Here's how the part is built. I have some questions about the finished solid (model axes, mm). A direction names the side the tool comes from. Give positions to 0.01 mm unless a question says otherwise; leave off trailing zeros. Loops run counter-clockwise (first coordinate to the right, second up) from the corner with the lowest first, then second, coordinate; pieces in that order, holes last.
Q1. Thinking about a two-plate mould opening in X: for faces 6 (the face through (-114, 50, -1)), 7 (the face through (111.01, 64.09, -2.66)), 8 (the face through (111.01, 114.09, -195.07)), which applies, pulls with the +X half, pulls with the -X half, needs draft (parallel to the pull), parting line crosses it, or undercut?
Q2. Suppose I cut it at D-D (y = 89). List the corners of the cut face in (x, z) for me.
Q3. Suppose I cut it at C-C (y = 139). List the corners of the cut face in (x, z) for me, and give its area (3 significant figures).
Q4. Suppose I cut it at B-B (x = -35.5). List the corners of the cut face in (y, z) for me, and give its area (3 significant figures).
Q5. Suppose I cut it at A-A (z = 9). List the corners of the cut face in (x, y) for me, and give its area (3 significant figures).
Q6. I need wall thicknesses on probe 1 along Z at (x, y) = (247, -67); probe 2 along Y at (x, z) = (243, 50); probe 3 along X at (y, z) = (-34, -64). Which ranges of each line are inside material? Lowest first, please.
Q7. For faces 1 (the face through (71, 70, -190)), 2 (the face through (237, 130, -3)), 3 (the face through (240.167, -65, 3)), 4 (the face through (99, 42, -200)), 5 (the face through (245, -100, 3)), which set-ups out of +Z, -Z, +X, -X, +Y, -Y let a thin tool reach every point of the face, with its end or its side?
Q8. I'm going to push flat-ended pins straight in: P1, Ø4, axis at x = 141.5, z = -69.5, coming from the +Y side; P2, Ø1, axis at y = 98.5, z = 80.5, coming from the -X side; P3, Ø1, axis at x = 157, z = -153, coming from the -Y side; P4, Ø11, axis at y = -67, z = -50, coming from the +X side. Where does each tip first touch, or does it pass through?
Autodesk Inventor part; units mm, degrees
ref_plane "Work Plane2" through (250.1666, 130, 0) normal (0, 0, -1) x (-1, 0, 0)
ref_plane "YZ Plane" through (0, 0, 0) normal (1, 0, 0) x (0, 1, 0)
ref_plane "XZ Plane" through (0, 0, 0) normal (0, 1, 0) x (-1, 0, 0)
sketch "Sketch1" plane through (0, 0, 0) normal (0, 0, 1) x (1, 0, 0)
  line L0 (0, 0) -> (225.1666, 130)
  line L1 (0, 0) -> (260, 0) construction
  line L2 (225.1666, 130) -> (250.1666, 130)
  line L3 (250.1666, 130) -> (250.1666, 0)
  line L4 (250.1666, 0) -> (0, 0)
  dimension "d4" = 30
  dimension "d5" = 260
  dimension "d6" = 25
extrude "Extrusion1" add sketch "Sketch1" along normal blind 200 and the other way blind 200
sketch "Sketch8" plane through (250.1666, 0, -200) normal (0, -1, 0) x (1, 0, 0)
  line L0 (0, 0) -> (-250.1666, 0)
  line L1 (0, 400) -> (0, 390)
  line L2 (-260.64, 0) -> (0, 0)
  line L3 (0, 0) -> (0, 400)
  line L4 (0, 400) -> (-260.64, 400)
  line L5 (-260.64, 400) -> (-260.64, 0)
  point P0 (-250.1666, 200)
extrude "Extrusion8" add sketch "Sketch8" along normal blind 30
sketch "Sketch9" plane through (-10.4734, -30, -200) normal (-1, 0, 0) x (0, 0, 1)
  line L0 (0, 160) -> (0, 0)
  line L1 (400, 160) -> (400, 0)
  line L2 (0, 0) -> (400, 0)
  line L3 (400, 0) -> (400, 30)
  line L4 (400, 30) -> (0, 30)
  line L5 (0, 30) -> (0, 0)
  point P0 (200, 30)
  point P1 (0, 229.8807)
  point P2 (400, 229.8807)
extrude "Extrusion9" add sketch "Sketch9" along normal blind 120
sketch "Sketch10" plane through (-130.4734, 0, -200) normal (0, 1, 0) x (1, 0, 0)
  line L0 (380.64, -400) -> (0, -400)
  line L1 (380.64, 0) -> (0, 0)
  line L2 (0, -400) -> (20, -400)
  line L3 (20, -400) -> (20, 0)
  line L4 (20, 0) -> (0, 0)
  line L5 (0, 0) -> (0, -400)
  point P0 (130.4734, -200)
  dimension "d32" = 20
extrude "Extrusion10" add sketch "Sketch10" along normal blind 50
sketch "Sketch11" plane through (0, 0, -200) normal (0, 0, -1) x (-1, 0, 0)
  line L0 (-250.1666, 130) -> (-250.1666, -30)
  line L1 (-250.1666, 130) -> (-250.1666, 180)
  line L2 (0, 0) -> (-225.1666, 130)
  line L3 (0, 0) -> (0, 50)
  line L4 (110.4734, 0) -> (110.4734, 50)
  line L5 (0, 50) -> (110.4734, 50)
  line L6 (0, 50) -> (-225.1666, 180)
  line L7 (-225.1666, 180) -> (-250.1666, 180)
  line L8 (-225.1666, 130) -> (-225.1666, 180)
  line L9 (-225.1666, 130) -> (-250.1666, 130)
  line L10 (0, 0) -> (110.4734, 0)
  dimension "d35" = 50
  dimension "d36" = 50
extrude "Extrusion11" add sketch "Sketch11" against normal blind 10
ref_plane "Work Plane2" through (250.1666, 130, 0) normal (0, 0, -1) x (-1, 0, 0)
ref_plane "Work Plane1" through (250.1666, 130, 5) normal (0, 0, -1) x (-1, 0, 0)
mirror "Mirror1" about plane through (250.1666, 130, 0) normal (0, 0, -1) of "Extrusion11"
sketch "Sketch12" plane through (250.1666, -30, -200) normal (0, -1, 0) x (1, 0, 0)
  line L0 (0, 400) -> (-380.64, 400)
  line L1 (0, 400) -> (-10, 400)
  line L2 (-10, 400) -> (-10, 0)
  line L3 (-10, 0) -> (0, 0)
  line L4 (0, 0) -> (0, 400)
  point P0 (-250.1666, 200)
  dimension "d40" = 10
extrude "Extrusion12" add sketch "Sketch12" along normal blind 70
sketch "Sketch13" plane through (240.1666, -30, -200) normal (-1, 0, 0) x (0, 0, 1)
  line L0 (0, 0) -> (0, -70)
  line L1 (0, 0) -> (400, 0)
  point P0 (200, 30)
  point P1 (50, -37)
  dimension "d43" = 50
  dimension "d44" = 37
hole "Hole1" at (240.1666, -67, -150) direction (1, 0, 0) diameter 8.376 depth 27.3 tip angle 118
pattern_linear "Rectangular Pattern1" count 4 spacing 100 along (0, 0, 1) of "Hole1"
properties part number "rampa"
Solutions:
1. face 6: needs draft
1. face 7: undercut
1. face 8: pulls with the -X half
2. outline: (67.55, -200) - (250.17, -200) - (250.17, 200) - (67.55, 200) - (67.55, 190) - (154.15, 190) - (154.15, -190) - (67.55, -190) - close
3. outline: (154.15, -200) - (250.17, -200) - (250.17, -190) - (154.15, -190) - close; (154.15, 190) - (250.17, 190) - (250.17, 200) - (154.15, 200) - close
3. area: 1,920 mm2
4. outline: (-30, -200) - (50, -200) - (50, -190) - (0, -190) - (0, 190) - (50, 190) - (50, 200) - (-30, 200) - close
4. area: 13,000 mm2
5. outline: (-130.47, -30) - (240.17, -30) - (240.17, -100) - (250.17, -100) - (250.17, 130) - (225.17, 130) - (0, 0) - (-110.47, 0) - (-110.47, 50) - (-130.47, 50) - close
5. area: 31,000 mm2
6. probe 1: z = -200 to -154.19, -145.81 to -54.19, -45.81 to 45.81, 54.19 to 145.81, 154.19 to 200
6. probe 2: y = -100 to -71.19, -62.81 to 130
6. probe 3: x = 240.17 to 250.17
7. face 1: +Y
7. face 2: +X, -X, +Y
7. face 3: +Z, -Z, -X, -Y
7. face 4: -Z, +X, -X, +Y, -Y
7. face 5: +Z, -Z, +X, -X, -Y
8. P1: stops at y = 82.85
8. P2: stops at x = 169.74
8. P3: stops at y = -30
8. P4: stops at x = 250.17
